```python
from build123d import *

# Parameters (mm, degrees)
F1_DEPTH = 39
F2_DEPTH = 50
F3_W     = 100
F3_H     = 50
F4_DEPTH = 150
F6_W     = 20
F6_H     = 19.5
F7_DEPTH = 76.8
F8_W     = 9
F8_H     = 19.5
F9_DEPTH = 617


with BuildPart() as f1:
    # F0 (on Top) → F1 (new body)
    with BuildSketch(Plane.XY):
        with BuildLine():
            ThreePointArc((45.8257569496, -20), (50, 0), (45.8257569496, 20))
            Line((45.8257569496, 20), (0, 20))
            Line((0, 20), (0, -20))
            Line((0, -20), (45.8257569496, -20))
        make_face()
    extrude(amount=F1_DEPTH)

    # F0 (on Top) → F2 (join)
    with BuildSketch(Plane.XY):
        with BuildLine():
            Line((150, -50), (150, 50))
            Line((150, 50), (40.307905525, 50))
            Line((40.307905525, 50), (40.307905525, 29.5850089098))
            ThreePointArc((40.307905525, 29.5850089098), (43.3326672589, 24.945539646), (45.8257569496, 20))
            ThreePointArc((45.8257569496, 20), (50, 0), (45.8257569496, -20))
            ThreePointArc((45.8257569496, -20), (43.3326672589, -24.945539646), (40.307905525, -29.5850089098))
            Line((40.307905525, -29.5850089098), (40.307905525, -50))
            Line((40.307905525, -50), (150, -50))
        make_face()
    extrude(amount=F2_DEPTH)

    # F3 (on face) → F4 (join)
    with BuildSketch(Plane.YZ.offset(150)):
        with Locations((0, 25)):
            Rectangle(F3_W, F3_H)
    extrude(amount=F4_DEPTH)

    # F5: F1 across plane


with BuildPart() as f1_1:
    add(f1.part)
    add(f1.part.mirror(Plane.YZ))

    # F6 (on Front) → F7 (cut, symmetric)
    with BuildSketch(Plane.XZ):
        with Locations((0, 29.25)):
            Rectangle(F6_W, F6_H)
    extrude(amount=F7_DEPTH, both=True, mode=Mode.SUBTRACT)

    # F8 (on face) → F9 (cut, symmetric)
    with BuildSketch(Plane.XZ.offset(20)):
        with Locations((14.5, 29.25)):
            Rectangle(F8_W, F8_H)
        with Locations((-14.5, 29.25)):
            Rectangle(F8_W, F8_H)
    extrude(amount=F9_DEPTH, both=True, mode=Mode.SUBTRACT)


solid = f1_1.part
```
Input: part model. Units: mm. Frame: model coordinates. A direction names the side the tool comes from. Round coordinates to 2 decimals unless told otherwise and drop trailing zeros. Loops run counter-clockwise (first coordinate to the right, second up) from the corner with the lowest first, then second, coordinate; pieces in that order, holes last. Notation, with made-up numbers: M 44,1 L 62,1 A27 cw 62,18 Z; hole C -4,-10 d8. An arc over 180 degrees is marked long. Answer in a Markdown table with one row per item. Add a question column.
1. Section D-D (x = 5). Output: boundary loops of the cut face in (y, z), and give its area (3 significant figures).
2. Ray query, probe 1 along X at (y, z) = (31, 20); probe 2 along X at (y, z) = (20, 41); probe 3 along Z at (x, y) = (17, 4.5). Return the intervals inside material, ascending.
3. Section B-B (z = 32). Output: boundary loops of the cut face in (x, y) (3 decimals), and give its area (3 significant figures).
4. Mould query, pull axis X, two halves, no side actions, for faces 6 (the face through (19, 0, 29)), 7 (the face through (300, -1, 25)), 8 (the face through (4, -1, 0)). Classes: released by +X, released by -X, zero draft, split by the parting line, or undercut.
5. Contact query for a flat-ended pin moving along its axis: pin 1 (11.5 mm diameter, centred on x = -8, y = -7, fed in from +Z). Output: stop coordinate, or through.
6. Section C-C (z = 8). Output: boundary loops of the cut face in (x, y) (3 decimals), and give its area (3 significant figures).
7. Section A-A (y = -39). Output: boundary loops of the cut face in (x, z), and give its area (3 significant figures).
8. Set-up query: faces 1 (the face through (1, -20, 19)), 2 (the face through (40.308, -40, 25)), 3 (the face through (40.308, 40, 25)), 4 (the face through (-19, 0, 29)), 5 (the face through (-34, 0, 39)). Return all of +Z, -Z, +X, -X, +Y, -Y with unobstructed straight access to the full face (end or side cutting, diameter ignored); none if empty.
Values follow:
| question | item | result |
|---|---|---|
| 1 | outline | M -20,0 L 20,0 L 20,19.5 L -20,19.5 Z |
| 1 | area | 780 mm^2 |
| 2 | probe 1 | -300 to -40.31, 40.31 to 300 |
| 2 | probe 2 | -300 to -45.83, 45.83 to 300 |
| 2 | probe 3 | 0 to 19.5 |
| 3 | outline | M -300,-50 L -40.308,-50 L -40.308,-29.585 A50 cw -45.826,-20 L -19,-20 L -19,20 L -45.826,20 A50 cw -40.308,29.585 L -40.308,50 L -300,50 Z; M 19,-20 L 45.826,-20 A50 cw 40.308,-29.585 L 40.308,-50 L 300,-50 L 300,50 L 40.308,50 L 40.308,29.585 A50 cw 45.826,20 L 19,20 Z |
| 3 | area | 53,500 mm^2 |
| 4 | face 6 | undercut |
| 4 | face 7 | released by +X |
| 4 | face 8 | zero draft |
| 5 | pin 1 | z = 19.5 |
| 6 | outline | M -300,-50 L -40.308,-50 L -40.308,-29.585 A50 cw -45.826,-20 L 45.826,-20 A50 cw 40.308,-29.585 L 40.308,-50 L 300,-50 L 300,50 L 40.308,50 L 40.308,29.585 A50 cw 45.826,20 L -45.826,20 A50 cw -40.308,29.585 L -40.308,50 L -300,50 Z |
| 6 | area | 55,000 mm^2 |
| 7 | outline | M -300,0 L -40.31,0 L -40.31,50 L -300,50 Z; M 40.31,0 L 300,0 L 300,50 L 40.31,50 Z |
| 7 | area | 26,000 mm^2 |
| 8 | face 1 | +Z, -Z |
| 8 | face 2 | +Z, -Z, -Y |
| 8 | face 3 | +Z, -Z, +Y |
| 8 | face 4 | +Z, +Y, -Y |
| 8 | face 5 | +Z |
